The drawing under review shows one solid part. Ordinate dimensions are in mm from its lowest x, y, z. Give positions to 0.01 mm unless a question says otherwise; leave off trailing zeros. Loops run counter-clockwise (first coordinate to the right, second up) from the corner with the lowest first, then second, coordinate; pieces in that order, holes last. Notation, with made-up numbers: (65.5, -31.5) - (102.5, -31.5) arc R8 cw to (102.5, -22.5) - close; hole circle Ø7 at (-19.5, 41). An arc over 180 degrees is marked (long way). Answer as CSV lines item,"result".
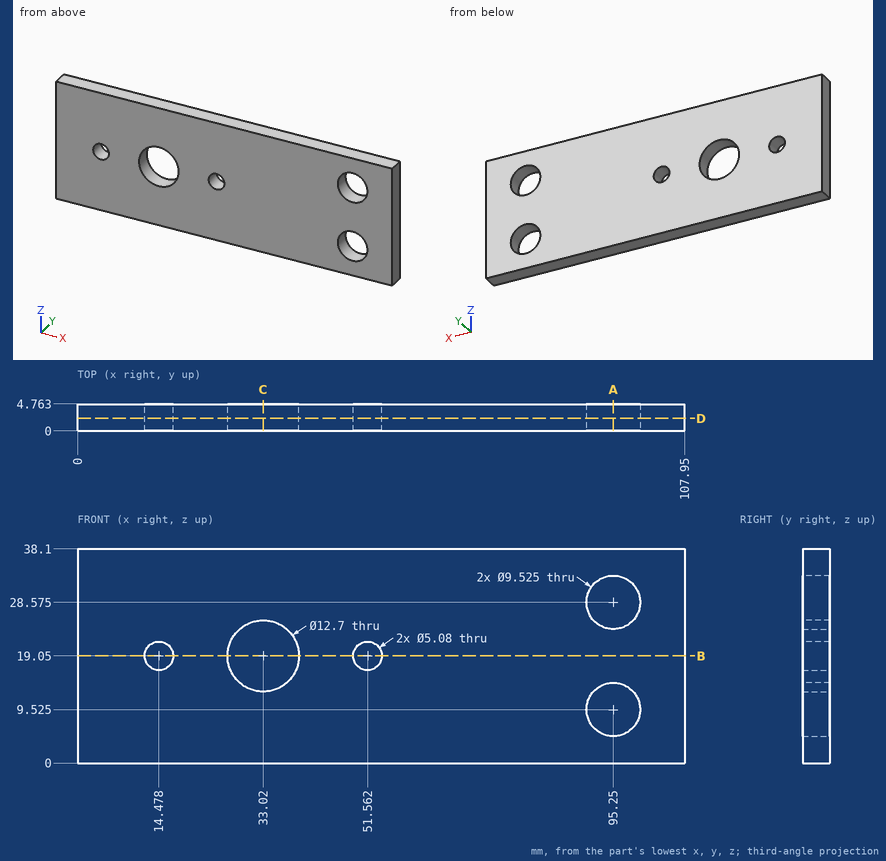
1) Consider section B-B on z = 19.05. Write out the cut boundary in (x, y), and give its area (3 significant figures).
From the geometry:
outline,"(0, 0) - (11.94, 0) - (11.94, 4.76) - (0, 4.76) - close; (17.02, 0) - (26.67, 0) - (26.67, 4.76) - (17.02, 4.76) - close; (39.37, 0) - (49.02, 0) - (49.02, 4.76) - (39.37, 4.76) - close; (54.1, 0) - (107.95, 0) - (107.95, 4.76) - (54.1, 4.76) - close"
area,"405 mm^2"
2) Consider section A-A on x = 95.25. Write out the cut boundary in (y, z).
From the geometry:
outline,"(0, 0) - (4.76, 0) - (4.76, 4.76) - (0, 4.76) - close; (0, 14.29) - (4.76, 14.29) - (4.76, 23.81) - (0, 23.81) - close; (0, 33.34) - (4.76, 33.34) - (4.76, 38.1) - (0, 38.1) - close"
3) Consider section C-C on x = 33.02. Write out the cut boundary in (y, z).
From the geometry:
outline,"(0, 0) - (4.76, 0) - (4.76, 12.7) - (0, 12.7) - close; (0, 25.4) - (4.76, 25.4) - (4.76, 38.1) - (0, 38.1) - close"
4) Wall thickness on line 1 (X direction, y = 2.1, z = 19.05); line 2 (Z direction, x = 97, y = 3.15) (1 decimal); line 3 (Z direction, x = 32, y = 3.5): over which ranges is each line inside the solid? List them lowest first. Write a range as from..to.
From the geometry:
line 1,"x = 0..11.94, 17.02..26.67, 39.37..49.02, 54.1..107.95"
line 2,"z = 0..5.1, 14..24.1, 33..38.1"
line 3,"z = 0..12.78, 25.32..38.1"
5) Consider section D-D on y = 2.2. Count the separate pieces of the cut face and the enclosed holes in it, and give its area (3 significant figures).
From the geometry:
separate pieces,"1"
enclosed holes,"5"
area,"3,800 mm^2"
